```python
from build123d import *

# Parameters (mm, degrees)
ESQUISSE1_W                = 355.6
ESQUISSE1_H                = 152.4
BOSS_EXTRU_1_DEPTH         = 6.35
ESQUISSE3_W                = 6.35
ESQUISSE3_H                = 25.4
ENL_V_MAT_EXTRU_2_DEPTH    = 6.35
R_P_TITION_LIN_AIRE2_COUNT = 3
R_P_TITION_LIN_AIRE2_PITCH = 50.8
SYM_TRIE1_COPY_1_SKETCH_W  = 6.35
SYM_TRIE1_COPY_1_SKETCH_H  = 25.4
SYM_TRIE1_COPY_1_DEPTH     = 6.35
SYM_TRIE1_COPY_2_SKETCH_W  = 6.35
SYM_TRIE1_COPY_2_SKETCH_H  = 25.4
SYM_TRIE1_COPY_2_DEPTH     = 6.35
CUT_EXTRUDE1_REACH         = 195.545
SKETCH1_W                  = 228.6
SKETCH1_H                  = 63.5
ESQUISSE5_W                = 38.1
ESQUISSE5_H                = 6.35
ENL_V_MAT_EXTRU_4_DEPTH    = 6.35
ESQUISSE6_W                = 25.4
ESQUISSE6_H                = 6.35
ENL_V_MAT_EXTRU_5_DEPTH    = 6.35
R_P_TITION_LIN_AIRE3_COUNT = 5
R_P_TITION_LIN_AIRE3_PITCH = 50.8
ESQUISSE8_W                = 12.7
ESQUISSE8_H                = 6.35
BOSS_EXTRU_2_DEPTH         = 6.35


with BuildPart() as part:
    # Esquisse1 → Boss.-Extru.1 (new body)
    with BuildSketch(Plane.XY):
        Rectangle(ESQUISSE1_W, ESQUISSE1_H)
    extrude(amount=BOSS_EXTRU_1_DEPTH)

    # Esquisse3 → Enlèv. mat.-Extru.2 (cut)
    with BuildSketch(Plane.XY.offset(6.35)):
        with Locations((-174.625, 50.8)):
            Rectangle(ESQUISSE3_W, ESQUISSE3_H)
    enl_v_mat_extru_2 = extrude(amount=-ENL_V_MAT_EXTRU_2_DEPTH, mode=Mode.SUBTRACT)

    # Répétition linéaire2: Enlèv. mat.-Extru.2 ×3
    with Locations(*[(0, -i * R_P_TITION_LIN_AIRE2_PITCH, 0) for i in range(1, R_P_TITION_LIN_AIRE2_COUNT)]):
        add(enl_v_mat_extru_2, mode=Mode.SUBTRACT)

    # Symétrie1: Enlèv. mat.-Extru.2 across plane
    add(enl_v_mat_extru_2.mirror(Plane(origin=(0, 0, 0), x_dir=(0, 0, 1), z_dir=(1, 0, 0))), mode=Mode.SUBTRACT)

    # Symétrie1 copy 1 sketch → Symétrie1 copy 1 (cut)
    with BuildSketch(Plane(origin=(0, -50.8, 6.35), x_dir=(-1, 0, 0), z_dir=(0, 0, 1))):
        with Locations((-174.625, -50.8)):
            Rectangle(SYM_TRIE1_COPY_1_SKETCH_W, SYM_TRIE1_COPY_1_SKETCH_H)
    extrude(amount=-SYM_TRIE1_COPY_1_DEPTH, mode=Mode.SUBTRACT)

    # Symétrie1 copy 2 sketch → Symétrie1 copy 2 (cut)
    with BuildSketch(Plane(origin=(0, -101.6, 6.35), x_dir=(-1, 0, 0), z_dir=(0, 0, 1))):
        with Locations((-174.625, -50.8)):
            Rectangle(SYM_TRIE1_COPY_2_SKETCH_W, SYM_TRIE1_COPY_2_SKETCH_H)
    extrude(amount=-SYM_TRIE1_COPY_2_DEPTH, mode=Mode.SUBTRACT)

    # Sketch1 → Cut-Extrude1 (cut, up to next)
    with BuildSketch(Plane.XY.offset(6.35), mode=Mode.PRIVATE) as cut_extrude1_sk1:
        with Locations((-38.1, -44.45)):
            Rectangle(SKETCH1_W, SKETCH1_H)
    cut_extrude1_tool1 = extrude(cut_extrude1_sk1.sketch, amount=-CUT_EXTRUDE1_REACH, mode=Mode.PRIVATE) & part.part
    add(cut_extrude1_tool1.solids().sort_by_distance((-38.1, -44.45, 6.35))[0], mode=Mode.SUBTRACT)

    # Esquisse5 → Enlèv. mat.-Extru.4 (cut)
    with BuildSketch(Plane.XY.offset(6.35)):
        with Locations((-158.75, 22.225)):
            Rectangle(ESQUISSE5_W, ESQUISSE5_H)
    enl_v_mat_extru_4 = extrude(amount=-ENL_V_MAT_EXTRU_4_DEPTH, mode=Mode.SUBTRACT)

    # Symétrie2: Enlèv. mat.-Extru.4 across plane
    add(enl_v_mat_extru_4.mirror(Plane(origin=(0, 0, 0), x_dir=(0, 0, 1), z_dir=(1, 0, 0))), mode=Mode.SUBTRACT)

    # Esquisse6 → Enlèv. mat.-Extru.5 (cut)
    with BuildSketch(Plane.XY.offset(6.35)):
        with Locations((-101.6, 22.225)):
            Rectangle(ESQUISSE6_W, ESQUISSE6_H)
    enl_v_mat_extru_5 = extrude(amount=-ENL_V_MAT_EXTRU_5_DEPTH, mode=Mode.SUBTRACT)

    # Répétition linéaire3: Enlèv. mat.-Extru.5 ×5
    with Locations(*[(i * R_P_TITION_LIN_AIRE3_PITCH, 0, 0) for i in range(1, R_P_TITION_LIN_AIRE3_COUNT)]):
        add(enl_v_mat_extru_5, mode=Mode.SUBTRACT)

    # Esquisse8 → Boss.-Extru.2 (add)
    with BuildSketch(Plane.XY.offset(6.35)):
        with Locations((-165.1, -79.375)):
            Rectangle(ESQUISSE8_W, ESQUISSE8_H)
        with Locations((88.9, -79.375)):
            Rectangle(ESQUISSE8_W, ESQUISSE8_H)
        with Locations((114.3, -79.375)):
            Rectangle(ESQUISSE8_W, ESQUISSE8_H)
        with Locations((139.7, -79.375)):
            Rectangle(ESQUISSE8_W, ESQUISSE8_H)
        with Locations((165.1, -79.375)):
            Rectangle(ESQUISSE8_W, ESQUISSE8_H)
    extrude(amount=-BOSS_EXTRU_2_DEPTH)


solid = part.part
```
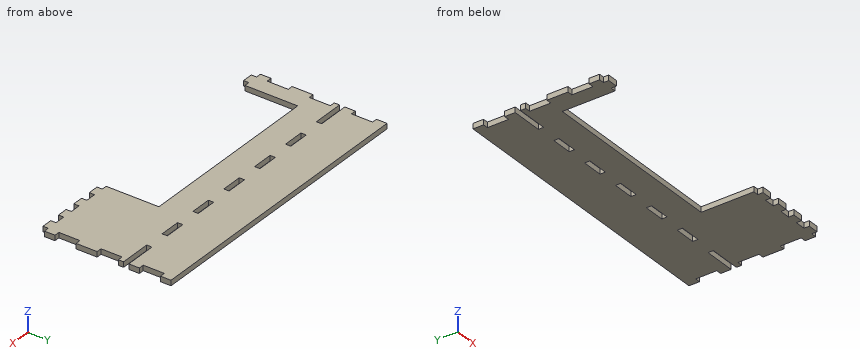
Read the model definition and answer for the solid it produces. Units are mm, in the model's axes. Give positions to 0.01 mm unless a question says otherwise; leave off trailing zeros. Write each loop counter-clockwise with the first axis right and the second up, starting at its lowest first coordinate (ties: lowest second). Pieces come first, ordered by that corner, then holes. Notation, with made-up numbers: (63, 8.25) - (103, 8.25) arc R29 ccw to (103, 30.25) - close; hole circle Ø7 at (43.25, 36). An arc over 180 degrees is marked (long way). Write item = value, one per line. Start each with the question number.
Item 1: Find the intervals of material crossed by probe 1 along Y at (x, z) = (144, 1); probe 2 along X at (y, z) = (-40.5, 0.75); probe 3 along Y at (x, z) = (-91, 1.5), in increasing order. Write a range as [from, to].
Item 2: Find section A-A (x = 150.5). Give the vertices of the cut face in (y, z), then the cut area to 3 significant figures.
Item 3: Each of these flat-tipped pins is pushed along its axis until it touches: P1, Ø1.9, axis at x = -174, z = 2.5, coming from the -Y side; P2, Ø8, axis at x = 72, y = -14, coming from the +Z side; P3, Ø3, axis at y = -79, z = 3, coming from the +X side; P4, Ø3, axis at y = 21.5, z = 4, coming from the +X side. Where does it stop, or does it pass through?
Item 4: Find section D-D (x = 34). Give the vertices of the cut face in (y, z), then the cut area to 3 significant figures.
Item 5: Find section B-B (y = -45.5). Give the vertices of the cut face in (x, z), then the cut area to 3 significant figures.
Item 6: Find section C-C (z = 1.5). State how many separate pieces and enclosed holes the cut face has, then the cut area to 3 significant figures.
Response:
q1.probe_1 = [-82.55, 19.05], [25.4, 76.2]
q1.probe_2 = [-171.45, -152.4], [76.2, 171.45]
q1.probe_3 = [-12.7, 19.05], [25.4, 76.2]
q2.outline = (-76.2, 0) - (19.05, 0) - (19.05, 6.35) - (-76.2, 6.35) - close; (25.4, 0) - (76.2, 0) - (76.2, 6.35) - (25.4, 6.35) - close
q2.area = 927 mm²
q3.P1 = -76.2
q3.P2 = 6.35
q3.P3 = 171.45
q3.P4 = 139.7
q4.outline = (-12.7, 0) - (76.2, 0) - (76.2, 6.35) - (-12.7, 6.35) - close
q4.area = 565 mm²
q5.outline = (-171.45, 0) - (-152.4, 0) - (-152.4, 6.35) - (-171.45, 6.35) - close; (76.2, 0) - (171.45, 0) - (171.45, 6.35) - (76.2, 6.35) - close
q5.area = 726 mm²
q6.separate_pieces = 1
q6.enclosed_holes = 5
q6.area = 37,800 mm²
